```python
from build123d import *

# Parameters (mm, degrees)
F0_W     = 65
F0_H     = 70
F0_W_2   = 11
F0_H_2   = 11
F1_DEPTH = 2.5


with BuildPart() as f1:
    # F0 (on Top) → F1 (new body)
    with BuildSketch(Plane.XY):
        with Locations((-12.392649, -0.425882)):
            Rectangle(F0_W, F0_H)
        with Locations((-34.892649, -22.925882)):
            Rectangle(F0_W_2, F0_H_2, mode=Mode.SUBTRACT)
        with Locations((-19.892649, -22.925882)):
            Rectangle(F0_W_2, F0_H_2, mode=Mode.SUBTRACT)
        with Locations((-34.892649, -7.925882)):
            Rectangle(F0_W_2, F0_H_2, mode=Mode.SUBTRACT)
        with Locations((-19.892649, -7.925882)):
            Rectangle(F0_W_2, F0_H_2, mode=Mode.SUBTRACT)
        with Locations((-4.892649, -22.925882)):
            Rectangle(F0_W_2, F0_H_2, mode=Mode.SUBTRACT)
        with Locations((10.107351, -22.925882)):
            Rectangle(F0_W_2, F0_H_2, mode=Mode.SUBTRACT)
        with Locations((-4.892649, -7.925882)):
            Rectangle(F0_W_2, F0_H_2, mode=Mode.SUBTRACT)
        with Locations((10.107351, -7.925882)):
            Rectangle(F0_W_2, F0_H_2, mode=Mode.SUBTRACT)
        with Locations((-34.892649, 7.074118)):
            Rectangle(F0_W_2, F0_H_2, mode=Mode.SUBTRACT)
        with Locations((-19.892649, 7.074118)):
            Rectangle(F0_W_2, F0_H_2, mode=Mode.SUBTRACT)
        with Locations((-34.892649, 22.074118)):
            Rectangle(F0_W_2, F0_H_2, mode=Mode.SUBTRACT)
        with Locations((-19.892649, 22.074118)):
            Rectangle(F0_W_2, F0_H_2, mode=Mode.SUBTRACT)
        with Locations((-4.892649, 7.074118)):
            Rectangle(F0_W_2, F0_H_2, mode=Mode.SUBTRACT)
        with Locations((10.107351, 7.074118)):
            Rectangle(F0_W_2, F0_H_2, mode=Mode.SUBTRACT)
        with Locations((-4.892649, 22.074118)):
            Rectangle(F0_W_2, F0_H_2, mode=Mode.SUBTRACT)
        with Locations((10.107351, 22.074118)):
            Rectangle(F0_W_2, F0_H_2, mode=Mode.SUBTRACT)
    extrude(amount=F1_DEPTH)


solid = f1.part
```
Here's how the part is built. I have some questions about the finished solid (model axes, mm). A direction names the side the tool comes from. Round coordinates to 2 decimals unless told otherwise and drop trailing zeros. Order: outer loops, then holes, each group sorted by start corner. A loop starts at its lowest first (then second) coordinate and runs counter-clockwise, first axis right, second up. Notation, with made-up numbers: (-5.5, 75.5) -> (50.5, 75.5) arc R22 cw to (50.5, 111.5) -> close; hole circle Ø2 at (1.25, 20.25). An arc over 180 degrees is marked (long way). Use a Markdown table: item, result. Add a question column.
(1) I need wall thicknesses on line 1 along Y through (x, z) = (-1, 1.7); line 2 along X through (y, z) = (-7.5, 0.3). Which ranges of each line are inside material? Lowest first, please.
(2) Suppose I cut it at A-A, the plane x = -30.5. Please give me the cut outline in (y, z), and give its area (3 significant figures).
(3) For faces 5 (the face through (-40.393, 22, 1)), 6 (the face through (-44.893, -1, 1)), which set-ups out of +Z, -Z, +X, -X, +Y, -Y let a thin tool reach every point of the face, with its end or its side?
(4) Suppose I cut it at B-B, the plane y = 25.5. Please give me the cut outline in (x, z), and give its area (3 significant figures).
(5) Suppose I cut it at C-C, the plane z = 1.7. Count the separate pieces of the cut face and the enclosed holes in it, and give its area (3 significant figures).
(6) If we mould it in two halves opening along Y, with no side actions, what happens to faces 1 (the face through (15.607, -23, 1)), 2 (the face through (-13, -35.426, 1)), 3 (the face through (-13, 34.574, 1)), 4 (the face through (20.107, -1, 1))? For each: released by +Y, released by -Y, zero draft, split by the parting line, or undercut.
(7) For pin 1 Ø1 at (x, y) = (-37, 26) entering from +Z, with a flat end and sliding along its axis, tell me the tip position at first contact or that it passes through.
Verdict:
| question | item | result |
|---|---|---|
| 1 | line 1 | -35.43 to -28.43, -17.43 to -13.43, -2.43 to 1.57, 12.57 to 16.57, 27.57 to 34.57 |
| 1 | line 2 | -44.89 to -40.39, -29.39 to -25.39, -14.39 to -10.39, 0.61 to 4.61, 15.61 to 20.11 |
| 2 | outline | (-35.43, 0) -> (-28.43, 0) -> (-28.43, 2.5) -> (-35.43, 2.5) -> close; (-17.43, 0) -> (-13.43, 0) -> (-13.43, 2.5) -> (-17.43, 2.5) -> close; (-2.43, 0) -> (1.57, 0) -> (1.57, 2.5) -> (-2.43, 2.5) -> close; (12.57, 0) -> (16.57, 0) -> (16.57, 2.5) -> (12.57, 2.5) -> close; (27.57, 0) -> (34.57, 0) -> (34.57, 2.5) -> (27.57, 2.5) -> close |
| 2 | area | 65.0 mm2 |
| 3 | face 5 | +Z, -Z |
| 3 | face 6 | +Z, -Z, -X, +Y, -Y |
| 4 | outline | (-44.89, 0) -> (-40.39, 0) -> (-40.39, 2.5) -> (-44.89, 2.5) -> close; (-29.39, 0) -> (-25.39, 0) -> (-25.39, 2.5) -> (-29.39, 2.5) -> close; (-14.39, 0) -> (-10.39, 0) -> (-10.39, 2.5) -> (-14.39, 2.5) -> close; (0.61, 0) -> (4.61, 0) -> (4.61, 2.5) -> (0.61, 2.5) -> close; (15.61, 0) -> (20.11, 0) -> (20.11, 2.5) -> (15.61, 2.5) -> close |
| 4 | area | 52.5 mm2 |
| 5 | separate pieces | 1 |
| 5 | enclosed holes | 16 |
| 5 | area | 2,610 mm2 |
| 6 | face 1 | undercut |
| 6 | face 2 | released by -Y |
| 6 | face 3 | released by +Y |
| 6 | face 4 | zero draft |
| 7 | pin 1 | through |
